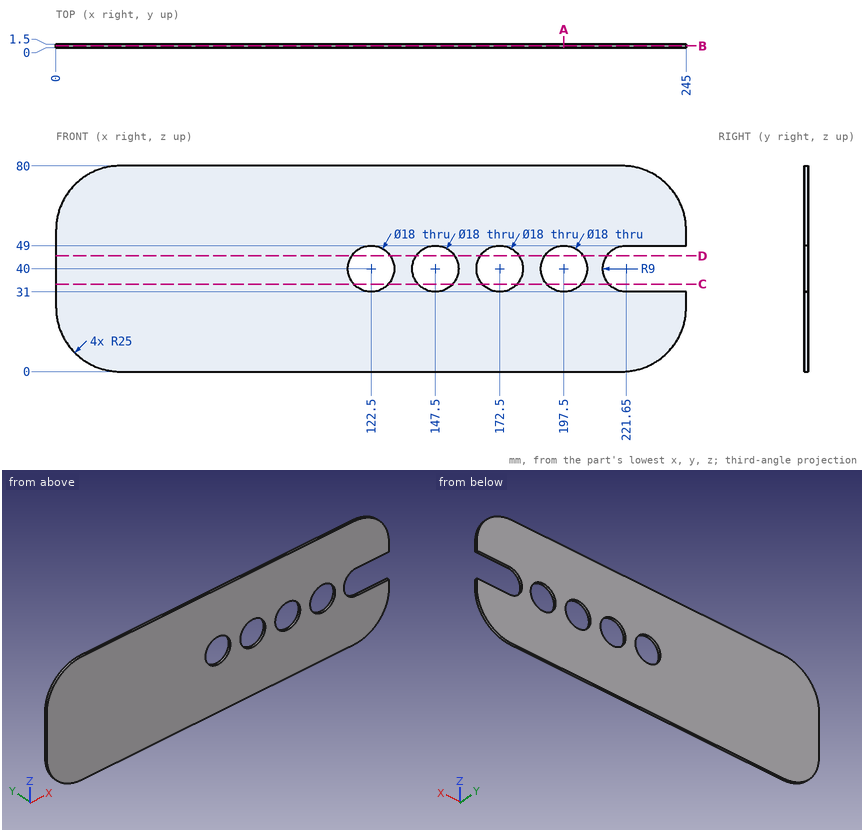
Study the drawing (mm; zero at the part's minimum x, y, z) and answer. Coordinates: 2 decimals unless noted, no trailing zeros. Order: outer loops, then holes, each group sorted by start corner. A loop starts at its lowest first (then second) coordinate and runs counter-clockwise, first axis right, second up. Notation, with made-up numbers: (4, -6) -> (20, -6) arc R20 ccw to (20, -2) -> close; hole circle Ø4 at (47, -25). An arc over 180 degrees is marked (long way). Answer in a Markdown table with one row per item. Add a question column.
Item 1: Find section B-B (y = 0.8). Write down the section's boundary in (x, z).
Item 2: Each of these flat-tipped pins is pushed along its axis until it touches: P1, Ø11, axis at x = 172.5, z = 40, coming from the +Y side; P2, Ø20.5, axis at x = 197.5, z = 40, coming from the +Y side; P3, Ø0.8, axis at x = 236, y = 0.5, coming from the +Z side. Where does it stop, or does it pass through?
Item 3: Find the intervals of material crossed by L1, parallel to X at y = 0.95, z = 40; L2, parallel to X at y = 0.7, z = 34; L3, parallel to Z at x = 205.5, y = 0.6, in increasing order. Write a range as from..to.
Item 4: Find section A-A (x = 197.5). Write down the section's boundary in (y, z).
Item 5: Find section C-C (z = 34). Write down the section's boundary in (x, y), then the cut area to 3 significant figures.
Item 6: Find section D-D (z = 45). Write down the section's boundary in (x, y).
Result set:
| question | item | result |
|---|---|---|
| 1 | outline | (0, 25) arc R25 ccw to (25, 0) -> (220, 0) arc R25 ccw to (245, 25) -> (245, 31) -> (221.65, 31) arc R9 cw to (221.65, 49) -> (245, 49) -> (245, 55) arc R25 ccw to (220, 80) -> (25, 80) arc R25 ccw to (0, 55) -> close; hole circle Ø18 at (122.5, 40); hole circle Ø18 at (147.5, 40); hole circle Ø18 at (172.5, 40); hole circle Ø18 at (197.5, 40) |
| 2 | P1 | passes through |
| 2 | P2 | stops at y = 1.5 |
| 2 | P3 | stops at z = 74.54 |
| 3 | L1 | x = 0..113.5, 131.5..138.5, 156.5..163.5, 181.5..188.5, 206.5..212.65 |
| 3 | L2 | x = 0..115.79, 129.21..140.79, 154.21..165.79, 179.21..190.79, 204.21..214.94 |
| 3 | L3 | z = 0..35.88, 44.12..80 |
| 4 | outline | (0, 0) -> (1.5, 0) -> (1.5, 31) -> (0, 31) -> close; (0, 49) -> (1.5, 49) -> (1.5, 80) -> (0, 80) -> close |
| 5 | outline | (0, 0) -> (115.79, 0) -> (115.79, 1.5) -> (0, 1.5) -> close; (129.21, 0) -> (140.79, 0) -> (140.79, 1.5) -> (129.21, 1.5) -> close; (154.21, 0) -> (165.79, 0) -> (165.79, 1.5) -> (154.21, 1.5) -> close; (179.21, 0) -> (190.79, 0) -> (190.79, 1.5) -> (179.21, 1.5) -> close; (204.21, 0) -> (214.94, 0) -> (214.94, 1.5) -> (204.21, 1.5) -> close |
| 5 | area | 242 mm² |
| 6 | outline | (0, 0) -> (115.02, 0) -> (115.02, 1.5) -> (0, 1.5) -> close; (129.98, 0) -> (140.02, 0) -> (140.02, 1.5) -> (129.98, 1.5) -> close; (154.98, 0) -> (165.02, 0) -> (165.02, 1.5) -> (154.98, 1.5) -> close; (179.98, 0) -> (190.02, 0) -> (190.02, 1.5) -> (179.98, 1.5) -> close; (204.98, 0) -> (214.17, 0) -> (214.17, 1.5) -> (204.98, 1.5) -> close |
